```python
from build123d import *

# Parameters (mm, degrees)
SKETCH_1_R          = 30
SKETCH_1_R_2        = 1.5
EXTRUDE_1_DEPTH     = 3
SKETCH_3_R          = 10
EXTRUDE_3_DEPTH     = 150
SKETCH_4_W          = 3
SKETCH_4_H          = 15
EXTRUDE_4_DEPTH     = 15
SKETCH_5_R          = 1.5
CUT_EXTRUDE_1_DEPTH = 175.51719113


with BuildPart() as part:
    # Эскиз1 → Бобышка-Вытянуть1 (new body)
    with BuildSketch(Plane.XY):
        Circle(SKETCH_1_R)
        with Locations((-20, 0)):
            Circle(SKETCH_1_R_2, mode=Mode.SUBTRACT)
        with Locations((0, -20)):
            Circle(SKETCH_1_R_2, mode=Mode.SUBTRACT)
        with Locations((20, 0)):
            Circle(SKETCH_1_R_2, mode=Mode.SUBTRACT)
        with Locations((0, 20)):
            Circle(SKETCH_1_R_2, mode=Mode.SUBTRACT)
    extrude(amount=EXTRUDE_1_DEPTH)

    # Эскиз3 → Бобышка-Вытянуть3 (add)
    with BuildSketch(Plane.XY.offset(3)):
        Circle(SKETCH_3_R)
    extrude(amount=EXTRUDE_3_DEPTH)

    # Эскиз4 → Бобышка-Вытянуть4 (add)
    with BuildSketch(Plane.XY.offset(153)):
        with Locations((-5, 0)):
            Rectangle(SKETCH_4_W, SKETCH_4_H)
        with Locations((5, 0)):
            Rectangle(SKETCH_4_W, SKETCH_4_H)
    extrude(amount=EXTRUDE_4_DEPTH)

    # Эскиз5 → Вырез-Вытянуть1 (cut, through all)
    with BuildSketch(Plane(origin=(6.5, 0, 0), x_dir=(0, 0, -1), z_dir=(1, 0, 0))):
        with Locations((-163, 0)):
            Circle(SKETCH_5_R)
    extrude(amount=-CUT_EXTRUDE_1_DEPTH, mode=Mode.SUBTRACT)


solid = part.part
```
Build history of the part. All positions in model axes, mm. A direction names the side the tool comes from. Give positions to 0.01 mm unless a question says otherwise; leave off trailing zeros. Loops run counter-clockwise (first coordinate to the right, second up) from the corner with the lowest first, then second, coordinate; pieces in that order, holes last. Notation, with made-up numbers: (-19.75, -10.5) -> (19.25, -10.5) arc R23 cw to (19.25, 11.5) -> close; hole circle Ø11 at (87, 15.25). An arc over 180 degrees is marked (long way). One line per question, with ' | ' between items.
Q1. Cut at B-B, the plane x = 24.5. Write the cut outline in (y, z).
Filled sheet:
outline: (-17.31, 0) -> (17.31, 0) -> (17.31, 3) -> (-17.31, 3) -> close
Q2. Drop flat-ended pins along their axis: pin 1 (1.5 mm diameter, centred on x = -5, z = 161.5, fed in from +Y); pin 2 (6 mm diameter, centred on x = 12, y = -19, fed in from +Z); pin 3 (5 mm diameter, centred on y = 0, z = 163, fed in from -X). Give the stop position or say it passes through.
Filled sheet:
pin 1: stops at y = 7.5 | pin 2: stops at z = 3 | pin 3: stops at x = -6.5
Q3. Pull direction Y, two halves, no side cores. Call faces 1 (the flat face through (5, 7.5, 160)), 2 (the cylindrical face through (-29.97, 1.32, 1.48)), 3 (the cylindrical face through (-4.979, -0.575, 161.614)): pulls with the +Y half, pulls with the -Y half, needs draft (parallel to the pull), parting line crosses it, or undercut.
Filled sheet:
face 1: pulls with the +Y half | face 2: parting line crosses it | face 3: undercut
Q4. Drill centre lines: line 1 along Y through (x, z) = (-5.65, 163); line 2 along Y through (x, z) = (0, 1); line 3 along Z through (x, y) = (23.5, 5.5). Where is each one in solid material? Low to high. Write a range as [from, to].
Filled sheet:
line 1: y = [-7.5, -1.5], [1.5, 7.5] | line 2: y = [-30, -21.5], [-18.5, 18.5], [21.5, 30] | line 3: z = [0, 3]
Q5. Cut at A-A, the plane z = 49. Write the cut outline in (x, y).
Filled sheet:
outline: circle Ø20 at (0, 0)
Q6. Tool access for faces 4 (the flat face through (5, -7.5, 160)), 5 (the flat face through (6.5, 0, 160)), 6 (the flat face through (-6.5, 0, 160)): list every direction of +Z, -Z, +X, -X, +Y, -Y with a clear straight run to the whole face (end or side of a thin tool).
Filled sheet:
face 4: +Z, +X, -X, -Y | face 5: +Z, +X, +Y, -Y | face 6: +Z, -X, +Y, -Y
Q7. Cut at C-C, the plane y = 15.5. Write the cut outline in (x, z).
Filled sheet:
outline: (-25.69, 0) -> (25.69, 0) -> (25.69, 3) -> (-25.69, 3) -> close
